```python
from build123d import *

# Parameters (mm, degrees)
CROQUIS1_W              = 30
CROQUIS1_H              = 14
SALIENTE_EXTRUIR1_DEPTH = 2.5
CROQUIS2_W              = 24.85
CROQUIS2_H              = 14
SALIENTE_EXTRUIR2_DEPTH = 20
CORTAR_EXTRUIR1_DEPTH   = 20


with BuildPart() as part:
    # Croquis1 → Saliente-Extruir1 (new body)
    with BuildSketch(Plane.XY):
        Rectangle(CROQUIS1_W, CROQUIS1_H)
    extrude(amount=SALIENTE_EXTRUIR1_DEPTH)

    # Croquis2 → Saliente-Extruir2 (add)
    with BuildSketch(Plane.XY.offset(2.5)):
        Rectangle(CROQUIS2_W, CROQUIS2_H)
    extrude(amount=SALIENTE_EXTRUIR2_DEPTH)

    # Croquis4 → Cortar-Extruir1 (cut)
    with BuildSketch(Plane(origin=(0, 7, 0), x_dir=(1, 0, 0), z_dir=(0, 1, 0))):
        Polygon((-12.425, -22.5), (0, -19.5), (12.425, -22.5), align=None)
    extrude(amount=-CORTAR_EXTRUIR1_DEPTH, mode=Mode.SUBTRACT)


solid = part.part
```
Geometry check sheet. Reference: the model listing, model coordinates, mm. A direction names the side the tool comes from. Coordinates: 2 decimals unless noted, no trailing zeros. Order: outer loops, then holes, each group sorted by start corner. A loop starts at its lowest first (then second) coordinate and runs counter-clockwise, first axis right, second up. Notation, with made-up numbers: (20, 14) - (55, 14) arc R15 cw to (55, 25) - close; hole circle Ø10 at (64.5, 51.25). An arc over 180 degrees is marked (long way). Answer in a Markdown table with one row per item. Add a question column.
1. Gauge pin test, flat ends, axial feed: pin 1 Ø1 at (y, z) = (1.5, 6.5) entering from +X (3 decimals); pin 2 Ø3 at (x, y) = (14.5, 3) entering from +Z; pin 3 Ø4 at (y, z) = (-0.5, 5.5) entering from -X (3 decimals). Record the tip position at first contact, or that the pin passes through.
2. Access from +Z, -Z, +X, -X, +Y, -Y to the whole of each face (thin tool, end or side, straight path). Record for faces 1 (the face through (12.425, 0, 12)), 2 (the face through (-14, 0, 2.5)), 3 (the face through (6.13, 0.1, 20.98)).
3. Draft check along X on faces 4 (the face through (-12.425, 0, 12)), 5 (the face through (-6.3, 0.1, 21.02)), 6 (the face through (15, 0, 1)). Enter one of: +X half, -X half, draft (parallel to the pull), parting line (faces both ways), or undercut.
4. Section check B-B (y = -4.25). Enter the section's corners in (x, z) (3 decimals).
5. Section check D-D (x = -7.75). Enter the section's corners in (y, z), plus the area to 3 significant figures.
6. Section check A-A (z = 20.25). Enter the section's corners in (x, y) (3 decimals), plus the area to 3 significant figures.
7. Material ranges on L1, parallel to X at y = -6, z = 2.75 (3 decimals); L2, parallel to Z at x = -13.5, y = -2.5; L3, parallel to Z at x = 8, y = 1.5, recorded low to high. Write a range as [from, to].
8. Section check C-C (z = 14.25). Enter the section's corners in (x, y) (3 decimals).
Data:
| question | item | result |
|---|---|---|
| 1 | pin 1 | stops at x = 12.425 |
| 1 | pin 2 | stops at z = 2.5 |
| 1 | pin 3 | stops at x = -12.425 |
| 2 | face 1 | +Z, +X, +Y, -Y |
| 2 | face 2 | +Z, -X, +Y, -Y |
| 2 | face 3 | +Z, +Y, -Y |
| 3 | face 4 | -X half |
| 3 | face 5 | undercut |
| 3 | face 6 | +X half |
| 4 | outline | (-15, 0) - (15, 0) - (15, 2.5) - (12.425, 2.5) - (12.425, 22.5) - (0, 19.5) - (-12.425, 22.5) - (-12.425, 2.5) - (-15, 2.5) - close |
| 5 | outline | (-7, 0) - (7, 0) - (7, 21.37) - (-7, 21.37) - close |
| 5 | area | 299 mm² |
| 6 | outline | (-12.425, -7) - (-3.106, -7) - (-3.106, 7) - (-12.425, 7) - close; (3.106, -7) - (12.425, -7) - (12.425, 7) - (3.106, 7) - close |
| 6 | area | 261 mm² |
| 7 | L1 | x = [-12.425, 12.425] |
| 7 | L2 | z = [0, 2.5] |
| 7 | L3 | z = [0, 21.43] |
| 8 | outline | (-12.425, -7) - (12.425, -7) - (12.425, 7) - (-12.425, 7) - close |
